Part model, mm, in its own coordinate system. A direction names the side the tool comes from. Give positions to 0.01 mm unless a question says otherwise; leave off trailing zeros. Write each loop counter-clockwise with the first axis right and the second up, starting at its lowest first coordinate (ties: lowest second). Pieces come first, ordered by that corner, then holes. Notation, with made-up numbers: M 59.25,75.5 L 74.25,75.5 A33 ccw 74.25,113.5 Z; hole C -33,0.5 d5. An arc over 180 degrees is marked long. Use CSV: the item, a comma, the result in double quotes. Start each with the question number.
1. Band-saw the part on A-A, the plane x = 111. List the corners of the cut face in (y, z).
2. Drop flat-ended pins along their axis: pin 1 Ø12 at (y, z) = (52.5, 45) entering from -X; pin 2 Ø1.5 at (x, z) = (99.5, -64) entering from +Y; pin 3 Ø3 at (x, y) = (-6, 50) entering from +Z. Give the stop position or say it passes through.
3. Mould opens along Y. For faces 1 (the face through (-5, 12, -54)), 2 (the face through (-2.465, 30.374, 47.641)), 3 (the face through (57.7, 36.7, 63.1)), 4 (the face through (57.68, -55.68, 32.56)) say: pulls with the +Y half, pulls with the -Y half, needs draft (parallel to the pull), parting line crosses it, or undercut.
4. 3-axis set-ups, long thin cutter, end or side, ignore diameter. For faces 5 (the face through (57.7, -0.4, -64.5)), 6 (the face through (0, 0, -57)), 7 (the face through (57.7, 0.4, 64.5)): which of +Z, -Z, +X, -X, +Y, -Y reach the whole face in a straight line?
5. Band-saw the part on B-B, the plane x = -8. List the corners of the cut face in (y, z), then the cut area to 3 significant figures.
6. Drill centre lines: line 1 along X through (y, z) = (59.5, -15); line 2 along X through (y, z) = (-40.5, 29); line 3 along Z through (x, y) = (149.5, -16). Where is each one in solid material? Low to high. Write a range as from..to.
from build123d import *

# Parameters (mm, degrees)
F0_R      = 56.5
F1_DEPTH  = 5
F2_R      = 55
F3_DEPTH  = 28.5
F5_DEPTH  = 117
F9_R      = 25
F10_DEPTH = 90


with BuildPart() as f1:
    # F0 (on Right) → F1 (new body)
    with BuildSketch(Plane.YZ):
        Circle(F0_R)
    extrude(amount=-F1_DEPTH)

    # F2 (on face) → F3 (join)
    with BuildSketch(Plane.YZ):
        Circle(F2_R)
    extrude(amount=-F3_DEPTH)

    # F4 (on Right) → F5 (join)
    with BuildSketch(Plane.YZ):
        with BuildLine():
            ThreePointArc((39.31518, 51.132833), (36.5, 63.219854), (24.624743, 59.614361))
            ThreePointArc((24.624743, 59.614361), (0, 64.5), (-24.624743, 59.614361))
            ThreePointArc((-24.624743, 59.614361), (-36.5, 63.219854), (-39.31518, 51.132833))
            ThreePointArc((-39.31518, 51.132833), (-55.858639, 32.25), (-63.939922, 8.481528))
            ThreePointArc((-63.939922, 8.481528), (-73, 0), (-63.939922, -8.481528))
            ThreePointArc((-63.939922, -8.481528), (-55.858639, -32.25), (-39.31518, -51.132833))
            ThreePointArc((-39.31518, -51.132833), (-36.5, -63.219854), (-24.624743, -59.614361))
            ThreePointArc((-24.624743, -59.614361), (0, -64.5), (24.624743, -59.614361))
            ThreePointArc((24.624743, -59.614361), (36.5, -63.219854), (39.31518, -51.132833))
            ThreePointArc((39.31518, -51.132833), (55.858639, -32.25), (63.939922, -8.481528))
            ThreePointArc((63.939922, -8.481528), (73, 0), (63.939922, 8.481528))
            ThreePointArc((63.939922, 8.481528), (55.858639, 32.25), (39.31518, 51.132833))
        make_face()
    extrude(amount=F5_DEPTH)

    # F6 (on Front) → F7 (revolve)
    with BuildSketch(Plane.XZ):
        with BuildLine():
            Line((142, 37), (142, 60.5))
            ThreePointArc((142, 60.5), (138.338835, 69.338835), (129.5, 73))
            Line((129.5, 73), (117, 73))
            Line((117, 73), (117, 0))
            Line((117, 0), (167, 0))
            Line((167, 0), (167, 37))
            Line((167, 37), (142, 37))
        make_face()
    revolve(axis=Axis((80.947809, 0, 0), (1, 0, 0)))

    # F9 (on face) → F10 (join)
    with BuildSketch(Plane(origin=(0, 0, 0), x_dir=(-1, 0, 0), z_dir=(0, 0.866025, 0.5))):
        with Locations((-142, -48)):
            Circle(F9_R)
    extrude(amount=-F10_DEPTH)


solid = f1.part
Output:
1,outline,"M -63.94,-8.48 A64.5 ccw -39.32,-51.13 A8.5 ccw long -24.62,-59.61 A64.5 ccw 24.62,-59.61 A8.5 ccw long 39.32,-51.13 A64.5 ccw 63.94,-8.48 A8.5 ccw long 63.94,8.48 A64.5 ccw 39.32,51.13 A8.5 ccw long 24.62,59.61 A64.5 ccw -24.62,59.61 A8.5 ccw long -39.32,51.13 A64.5 ccw -63.94,8.48 A8.5 ccw long Z"
2,pin 1,"stops at x = 0"
2,pin 2,"stops at y = 36.45"
2,pin 3,"stops at z = 28.33"
3,face 1,"needs draft"
3,face 2,"parting line crosses it"
3,face 3,"undercut"
3,face 4,"pulls with the -Y half"
4,face 5,"-Z, -X"
4,face 6,"-X"
4,face 7,"+Z, -X"
5,outline,"C 0,0 d110"
5,area,"9,500 mm²"
6,line 1,"x = 0..141.97"
6,line 2,"x = -28.5..142"
6,line 3,"z = -92.2..-37.13, -33.36..33.36"
